Geometry: final body of the model. Coordinates: model frame, mm. A direction names the side the tool comes from. Round coordinates to 2 decimals unless told otherwise and drop trailing zeros. Write each loop counter-clockwise with the first axis right and the second up, starting at its lowest first coordinate (ties: lowest second). Pieces come first, ordered by that corner, then holes. Notation, with made-up numbers: (72, 9) - (128, 9) arc R14 ccw to (128, 21) - close; hole circle Ø7 at (22, 73). An arc over 180 degrees is marked (long way). Use a Markdown table: item, result. Add a question column.
```python
from build123d import *

# Parameters (mm, degrees)
SKETCH1_W           = 38.1
SKETCH1_H           = 25.4
SKETCH1_W_2         = 31.75
SKETCH1_H_2         = 19.05
BOSS_EXTRUDE1_DEPTH = 558.8
CUT_EXTRUDE1_REACH  = 561.701
SKETCH2_R           = 4.7625
SKETCH2_R_2         = 2.54
SKETCH3_R           = 3.175
CUT_EXTRUDE2_DEPTH  = 3.175
SKETCH4_R           = 6.35
CUT_EXTRUDE3_DEPTH  = 3.175


with BuildPart() as part:
    # Sketch1 → Boss-Extrude1 (new body)
    with BuildSketch(Plane.XY):
        Rectangle(SKETCH1_W, SKETCH1_H)
        Rectangle(SKETCH1_W_2, SKETCH1_H_2, mode=Mode.SUBTRACT)
    extrude(amount=BOSS_EXTRUDE1_DEPTH)

    # Cut-Extrude1: up to this face of the body (flat: up to its plane)
    cut_extrude1_end = Plane(part.part.faces().sort_by_distance((0, -12.7, 279.4))[0])
    # Sketch2 → Cut-Extrude1 (cut, up to the picked face)
    with BuildSketch(Plane(origin=(0, 12.7, 0), x_dir=(1, 0, 0), z_dir=(0, 1, 0)), mode=Mode.PRIVATE) as cut_extrude1_sk1:
        with Locations(Location((0, -26.9875, 0), (0, 0, 270))):
            Circle(SKETCH2_R)
    cut_extrude1_tool1 = split(extrude(cut_extrude1_sk1.sketch, amount=-CUT_EXTRUDE1_REACH, mode=Mode.PRIVATE), bisect_by=cut_extrude1_end, keep=Keep.BOTH, mode=Mode.PRIVATE)
    # Sketch2 → Cut-Extrude1 (cut, up to the picked face)
    with BuildSketch(Plane(origin=(0, 12.7, 0), x_dir=(1, 0, 0), z_dir=(0, 1, 0)), mode=Mode.PRIVATE) as cut_extrude1_sk2:
        with Locations(Location((11.90625, -47.609729928, 0), (0, 0, 270))):
            Circle(SKETCH2_R_2)
    cut_extrude1_tool2 = split(extrude(cut_extrude1_sk2.sketch, amount=-CUT_EXTRUDE1_REACH, mode=Mode.PRIVATE), bisect_by=cut_extrude1_end, keep=Keep.BOTH, mode=Mode.PRIVATE)
    # Sketch2 → Cut-Extrude1 (cut, up to the picked face)
    with BuildSketch(Plane(origin=(0, 12.7, 0), x_dir=(1, 0, 0), z_dir=(0, 1, 0)), mode=Mode.PRIVATE) as cut_extrude1_sk3:
        with Locations(Location((-11.90625, -47.609729928, 0), (0, 0, 270))):
            Circle(SKETCH2_R_2)
    cut_extrude1_tool3 = split(extrude(cut_extrude1_sk3.sketch, amount=-CUT_EXTRUDE1_REACH, mode=Mode.PRIVATE), bisect_by=cut_extrude1_end, keep=Keep.BOTH, mode=Mode.PRIVATE)
    # Sketch2 → Cut-Extrude1 (cut, up to the picked face)
    with BuildSketch(Plane(origin=(0, 12.7, 0), x_dir=(1, 0, 0), z_dir=(0, 1, 0)), mode=Mode.PRIVATE) as cut_extrude1_sk4:
        with Locations(Location((-11.90625, -6.365270072, 0), (0, 0, 270))):
            Circle(SKETCH2_R_2)
    cut_extrude1_tool4 = split(extrude(cut_extrude1_sk4.sketch, amount=-CUT_EXTRUDE1_REACH, mode=Mode.PRIVATE), bisect_by=cut_extrude1_end, keep=Keep.BOTH, mode=Mode.PRIVATE)
    # Sketch2 → Cut-Extrude1 (cut, up to the picked face)
    with BuildSketch(Plane(origin=(0, 12.7, 0), x_dir=(1, 0, 0), z_dir=(0, 1, 0)), mode=Mode.PRIVATE) as cut_extrude1_sk5:
        with Locations(Location((11.90625, -6.365270072, 0), (0, 0, 270))):
            Circle(SKETCH2_R_2)
    cut_extrude1_tool5 = split(extrude(cut_extrude1_sk5.sketch, amount=-CUT_EXTRUDE1_REACH, mode=Mode.PRIVATE), bisect_by=cut_extrude1_end, keep=Keep.BOTH, mode=Mode.PRIVATE)
    add(cut_extrude1_tool1.solids().sort_by(Axis((0, 12.7, 26.9875), (0, -1, 0)))[0], mode=Mode.SUBTRACT)
    add(cut_extrude1_tool2.solids().sort_by(Axis((11.90625, 12.7, 47.60973), (0, -1, 0)))[0], mode=Mode.SUBTRACT)
    add(cut_extrude1_tool3.solids().sort_by(Axis((-11.90625, 12.7, 47.60973), (0, -1, 0)))[0], mode=Mode.SUBTRACT)
    add(cut_extrude1_tool4.solids().sort_by(Axis((-11.90625, 12.7, 6.36527), (0, -1, 0)))[0], mode=Mode.SUBTRACT)
    add(cut_extrude1_tool5.solids().sort_by(Axis((11.90625, 12.7, 6.36527), (0, -1, 0)))[0], mode=Mode.SUBTRACT)

    # Sketch3 → Cut-Extrude2 (cut)
    with BuildSketch(Plane.ZY.offset(19.05)):
        with Locations((538.1625, 0)):
            Circle(SKETCH3_R)
        with Locations((223.8375, 0)):
            Circle(SKETCH3_R)
    extrude(amount=-CUT_EXTRUDE2_DEPTH, mode=Mode.SUBTRACT)

    # Sketch4 → Cut-Extrude3 (cut)
    with BuildSketch(Plane(origin=(19.05, 0, 0), x_dir=(0, 0, -1), z_dir=(1, 0, 0))):
        with Locations((-223.8375, 0)):
            Circle(SKETCH4_R)
        with Locations((-538.1625, 0)):
            Circle(SKETCH4_R)
    extrude(amount=-CUT_EXTRUDE3_DEPTH, mode=Mode.SUBTRACT)


solid = part.part
```
1) Pin query (flat end, axial travel): P1, Ø4.5, axis at x = -11.91, z = 47.61, coming from the +Y side; P2, Ø8, axis at x = 3.5, y = -8, coming from the +Z side. Return the tip coordinate at first contact, or that it passes through.
2) Section A-A, the plane x = 0. Return the cut outline in (y, z) (3 decimals).
3) Set-up query: faces 1 (the cylindrical face through (17.485, 1.907, 532.106)), 2 (the flat face through (19.05, 0, 275)), 3 (the flat face through (15.875, 0, 275)). Return all of +Z, -Z, +X, -X, +Y, -Y with unobstructed straight access to the full face (end or side cutting, diameter ignored); none if empty.
4) Section B-B, the plane z = 345.5. Return the cut outline in (x, y) (3 decimals).
5) Draft query along Z for faces 4 (the flat face through (0, -11, 0)), 5 (the flat face through (0, -9.525, 275)), 6 (the cylindrical face through (0.21, -11.09, 22.23)). Return one class per face: released by +Z, released by -Z, zero draft, split by the parting line, or undercut.
6) Material intervals for L1, parallel to X at y = 7.75, z = 386 (3 decimals); L2, parallel to Y at x = 10, z = 392 (3 decimals); L3, parallel to Z at x = -17, y = 1, sorted ascending. Write a range as from..to.
Output values:
| question | item | result |
|---|---|---|
| 1 | P1 | passes through |
| 1 | P2 | stops at z = 558.8 |
| 2 | outline | (-12.7, 0) - (-9.525, 0) - (-9.525, 22.225) - (-12.7, 22.225) - close; (-12.7, 31.75) - (-9.525, 31.75) - (-9.525, 558.8) - (-12.7, 558.8) - close; (9.525, 0) - (12.7, 0) - (12.7, 22.225) - (9.525, 22.225) - close; (9.525, 31.75) - (12.7, 31.75) - (12.7, 558.8) - (9.525, 558.8) - close |
| 3 | face 1 | +X |
| 3 | face 2 | +Z, -Z, +X, +Y, -Y |
| 3 | face 3 | +Z, -Z |
| 4 | outline | (-19.05, -12.7) - (19.05, -12.7) - (19.05, 12.7) - (-19.05, 12.7) - close; hole (-15.875, -9.525) - (15.875, -9.525) - (15.875, 9.525) - (-15.875, 9.525) - close |
| 5 | face 4 | released by -Z |
| 5 | face 5 | zero draft |
| 5 | face 6 | undercut |
| 6 | L1 | x = -19.05..-15.875, 15.875..19.05 |
| 6 | L2 | y = -12.7..-9.525, 9.525..12.7 |
| 6 | L3 | z = 0..220.82, 226.85..535.15, 541.18..558.8 |
